Check sheet for the drawn part. Datum: minimum x, y, z corner. Units: mm. Give positions to 0.01 mm unless a question says otherwise; leave off trailing zeros. Loops run counter-clockwise (first coordinate to the right, second up) from the corner with the lowest first, then second, coordinate; pieces in that order, holes last. Notation, with made-up numbers: (-6.75, 33.25) - (12.25, 33.25) arc R19 ccw to (12.25, 43.25) - close; hole circle Ø8 at (63.25, 46.5). An arc over 180 degrees is marked (long way). Use one line per item in the form item = value.
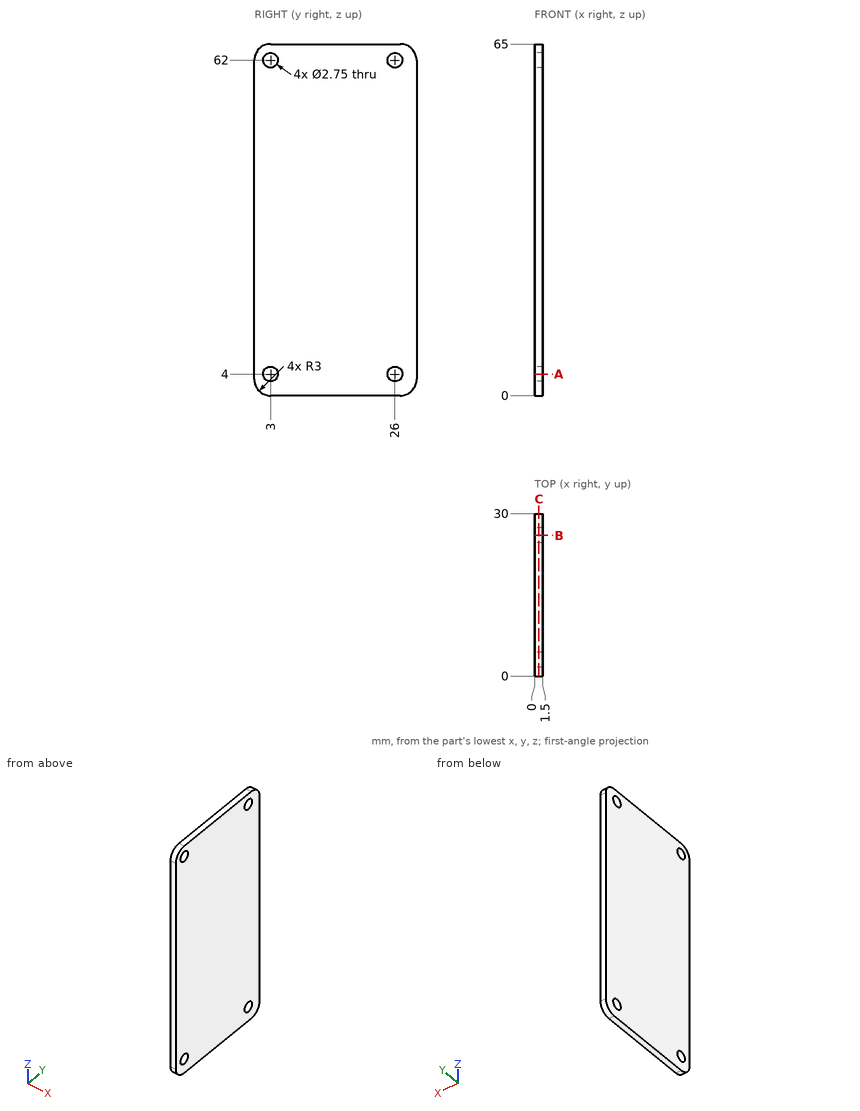
1. Section check B-B, the plane y = 26. Record the cut outline in (x, z) (3 decimals), then the cut area to 4 significant figures.
Result set:
outline = (0, 0) - (1.5, 0) - (1.5, 2.625) - (0, 2.625) - close; (0, 5.375) - (1.5, 5.375) - (1.5, 60.625) - (0, 60.625) - close; (0, 63.375) - (1.5, 63.375) - (1.5, 65) - (0, 65) - close
area = 89.25 mm²
2. Depth check by flat-ended pin: pin 1 Ø1.6 at (y, z) = (26, 62) entering from +X. Enter the tip coordinate at first touch or a pass-through.
Result set:
pin_1 = through
3. Section check C-C, the plane x = 0.8. Record the cut outline in (y, z) (3 decimals).
Result set:
outline = (0, 3) arc R3 ccw to (3, 0) - (27, 0) arc R3 ccw to (30, 3) - (30, 62) arc R3 ccw to (27, 65) - (3, 65) arc R3 ccw to (0, 62) - close; hole circle Ø2.75 at (3, 4); hole circle Ø2.75 at (3, 62); hole circle Ø2.75 at (26, 4); hole circle Ø2.75 at (26, 62)
4. Section check A-A, the plane z = 4. Record the cut outline in (x, y) (3 decimals), then the cut area to 4 significant figures.
Result set:
outline = (0, 0) - (1.5, 0) - (1.5, 1.625) - (0, 1.625) - close; (0, 4.375) - (1.5, 4.375) - (1.5, 24.625) - (0, 24.625) - close; (0, 27.375) - (1.5, 27.375) - (1.5, 30) - (0, 30) - close
area = 36.75 mm²
5. Scan lines: probe 1 along Y at (x, z) = (0.55, 4) (3 decimals); probe 2 along Z at (x, y) = (0.95, 3) (3 decimals); probe 3 along Y at (x, z) = (0.6, 3). Record each from-to range of solid material in increasing order.
Result set:
probe_1 = 0 to 1.625, 4.375 to 24.625, 27.375 to 30
probe_2 = 0 to 2.625, 5.375 to 60.625, 63.375 to 65
probe_3 = 0 to 2.06, 3.94 to 25.06, 26.94 to 30
